from build123d import *

# Parameters (mm, degrees)
F1_DEPTH = 2.8702
F3_DEPTH = 0.8382
F4_R     = 0.127
F7_SIZE  = 0.635


with BuildPart() as f1:
    # F0 (on Front) → F1 (new body, symmetric)
    with BuildSketch(Plane.XZ):
        with BuildLine():
            Line((10.935379, 11.6078), (0.964201, 11.6078))
            ThreePointArc((0.964201, 11.6078), (8.511631, 0), (0.964201, -11.6078))
            Line((0.964201, -11.6078), (10.951463, -11.6078))
            ThreePointArc((10.951463, -11.6078), (14.342647, -7.694951), (16.055431, -2.808553))
            Line((16.055431, -2.808553), (16.055431, 6.221704))
            ThreePointArc((16.055431, 6.221704), (13.874424, 9.275049), (10.935379, 11.6078))
        make_face()
    extrude(amount=F1_DEPTH, both=True)

    # F2 (on Front) → F3 (cut, symmetric)
    with BuildSketch(Plane.XZ):
        with BuildLine():
            ThreePointArc((6.826302, 11.6078), (11.813631, 0), (6.826302, -11.6078))
            Line((6.826302, -11.6078), (10.951463, -11.6078))
            ThreePointArc((10.951463, -11.6078), (14.342647, -7.694951), (16.055431, -2.808553))
            Line((16.055431, -2.808553), (16.055431, 6.221704))
            ThreePointArc((16.055431, 6.221704), (13.874424, 9.275049), (10.935379, 11.6078))
            Line((10.935379, 11.6078), (6.826302, 11.6078))
        make_face()
    extrude(amount=F3_DEPTH, both=True, mode=Mode.SUBTRACT)

    # F4
    f4_edges = [f1.edges().sort_by_distance(p)[0] for p in [
        (11.813631, 0.8382, 0),
        (11.813631, -0.8382, 0),
    ]]
    fillet(f4_edges, radius=F4_R)

    # F5 (on Top) → F6 (revolve, cut)
    with BuildSketch(Plane.XY):
        with BuildLine():
            Line((9.46572, 2.8702), (0.964201, 2.8702))
            Line((0.964201, 2.8702), (0.964201, -2.8702))
            Line((0.964201, -2.8702), (9.46572, -2.8702))
            ThreePointArc((9.46572, -2.8702), (9.339917, -2.69481), (9.222168, -2.513915))
            ThreePointArc((9.222168, -2.513915), (9.116906, -2.335376), (9.01949, -2.152438))
            ThreePointArc((9.01949, -2.152438), (8.930418, -1.966139), (8.849484, -1.776164))
            ThreePointArc((8.849484, -1.776164), (8.777234, -1.583993), (8.713312, -1.388894))
            ThreePointArc((8.713312, -1.388894), (8.658256, -1.192864), (8.611607, -0.994664))
            ThreePointArc((8.611607, -0.994664), (8.573786, -0.796647), (8.544357, -0.59721))
            ThreePointArc((8.544357, -0.59721), (8.52352, -0.398479), (8.511016, -0.19905))
            ThreePointArc((8.511016, -0.19905), (8.506865, 0), (8.511016, 0.19905))
            ThreePointArc((8.511016, 0.19905), (8.52352, 0.398479), (8.544357, 0.59721))
            ThreePointArc((8.544357, 0.59721), (8.573786, 0.796647), (8.611607, 0.994664))
            ThreePointArc((8.611607, 0.994664), (8.658256, 1.192864), (8.713312, 1.388894))
            ThreePointArc((8.713312, 1.388894), (8.777234, 1.583993), (8.849484, 1.776164))
            ThreePointArc((8.849484, 1.776164), (8.930418, 1.966139), (9.01949, 2.152438))
            ThreePointArc((9.01949, 2.152438), (9.116906, 2.335376), (9.222168, 2.513915))
            ThreePointArc((9.222168, 2.513915), (9.339917, 2.69481), (9.46572, 2.8702))
        make_face()
        with BuildLine():
            Line((9.322597, 2.286), (9.222168, 2.513915))
            ThreePointArc((9.222168, 2.513915), (9.116906, 2.335376), (9.01949, 2.152438))
            Line((9.01949, 2.152438), (9.322597, 2.286))
        make_face()
        with BuildLine():
            Line((9.138426, 1.932211), (9.01949, 2.152438))
            ThreePointArc((9.01949, 2.152438), (8.930418, 1.966139), (8.849484, 1.776164))
            Line((8.849484, 1.776164), (9.138426, 1.932211))
        make_face()
        with BuildLine():
            ThreePointArc((9.01949, -2.152438), (9.116906, -2.335376), (9.222168, -2.513915))
            Line((9.222168, -2.513915), (9.322597, -2.286))
            Line((9.322597, -2.286), (9.01949, -2.152438))
        make_face()
        with BuildLine():
            Line((8.985791, 1.563716), (8.849484, 1.776164))
            ThreePointArc((8.849484, 1.776164), (8.777234, 1.583993), (8.713312, 1.388894))
            Line((8.713312, 1.388894), (8.985791, 1.563716))
        make_face()
        with BuildLine():
            ThreePointArc((8.849484, -1.776164), (8.930418, -1.966139), (9.01949, -2.152438))
            Line((9.01949, -2.152438), (9.138426, -1.932211))
            Line((9.138426, -1.932211), (8.849484, -1.776164))
        make_face()
        with BuildLine():
            Line((8.865852, 1.183321), (8.713312, 1.388894))
            ThreePointArc((8.713312, 1.388894), (8.658256, 1.192864), (8.611607, 0.994664))
            Line((8.611607, 0.994664), (8.865852, 1.183321))
        make_face()
        with BuildLine():
            ThreePointArc((8.713312, -1.388894), (8.777234, -1.583993), (8.849484, -1.776164))
            Line((8.849484, -1.776164), (8.985791, -1.563716))
            Line((8.985791, -1.563716), (8.713312, -1.388894))
        make_face()
        with BuildLine():
            Line((8.779524, 0.793919), (8.611607, 0.994664))
            ThreePointArc((8.611607, 0.994664), (8.573786, 0.796647), (8.544357, 0.59721))
            Line((8.544357, 0.59721), (8.779524, 0.793919))
        make_face()
        with BuildLine():
            ThreePointArc((8.611607, -0.994664), (8.658256, -1.192864), (8.713312, -1.388894))
            Line((8.713312, -1.388894), (8.865852, -1.183321))
            Line((8.865852, -1.183321), (8.611607, -0.994664))
        make_face()
        with BuildLine():
            Line((8.727463, 0.398476), (8.544357, 0.59721))
            ThreePointArc((8.544357, 0.59721), (8.52352, 0.398479), (8.511016, 0.19905))
            Line((8.511016, 0.19905), (8.727463, 0.398476))
        make_face()
        with BuildLine():
            ThreePointArc((8.544357, -0.59721), (8.573786, -0.796647), (8.611607, -0.994664))
            Line((8.611607, -0.994664), (8.779524, -0.793919))
            Line((8.779524, -0.793919), (8.544357, -0.59721))
        make_face()
        with BuildLine():
            Line((8.710065, 0), (8.511016, 0.19905))
            ThreePointArc((8.511016, 0.19905), (8.506865, 0), (8.511016, -0.19905))
            Line((8.511016, -0.19905), (8.710065, 0))
        make_face()
        with BuildLine():
            ThreePointArc((8.511016, -0.19905), (8.52352, -0.398479), (8.544357, -0.59721))
            Line((8.544357, -0.59721), (8.727463, -0.398476))
            Line((8.727463, -0.398476), (8.511016, -0.19905))
        make_face()
    revolve(axis=Axis((-4.188369, -0.221392, 0), (0, -1, 0)), mode=Mode.SUBTRACT)

    # F7
    f7_edges = [f1.edges().sort_by_distance(p)[0] for p in [
        (16.055431, -0.8382, 1.706576),
        (16.055431, 0.8382, 1.706576),
    ]]
    chamfer(f7_edges, length=F7_SIZE)


solid = f1.part
Design review of the part built by this model. Coordinates are the model's own, in mm. A direction names the side the tool comes from. Round coordinates to 2 decimals unless told otherwise and drop trailing zeros. Loops run counter-clockwise (first coordinate to the right, second up) from the corner with the lowest first, then second, coordinate; pieces in that order, holes last. Notation, with made-up numbers: (-20, -10.75) - (3, -10.75) arc R17 cw to (3, -3.75) - close; hole circle Ø7 at (82.5, 82). An arc over 180 degrees is marked (long way). One line per item, written item: value. Start each with the question number.
1) To check wall thickness, follow L1, parallel to Y at x = 12.5, z = 0.5; L2, parallel to Z at x = 7, y = -1.75; L3, parallel to Z at x = 7, y = 0.1. State the ranges of each line that lie inside material, in increasing order. Write a range as from..to.
2) For faces 5 (the flat face through (12.1, -0.838, 0.2)), 6 (the flat face through (16.055, 2, 2)), list the 3-axis set-ups (+Z, -Z, +X, -X, +Y, -Y) from which the entire face can be reached by the end or side of a thin tool; tool diameter is ignored.
3) Draft analysis for pull direction Z (two halves, no side actions). For faces 1 (the flat face through (11, 2.87, 0)), 2 (the flat face through (6, 0, -11.608)), 3 (the conical face through (8.659, -0.694, -0.206)), 4 (the conical face through (8.74, -1.09, -0.21)), state which applies: +Z half, -Z half, draft (parallel to the pull), parting line (faces both ways), or undercut.
4) Consider section A-A on x = 12.25. Give the boundary of the cut face in (y, z), then the cut area to 3 significant figures.
Reported:
1. L1: y = -2.87..-0.84, 0.84..2.87
1. L2: z = -11.61..-6.73, 6.73..11.61
1. L3: z = -11.44..-6.21, 6.21..11.44
2. face 5: +X
2. face 6: +Z, -Z, +X, +Y, -Y
3. face 1: draft
3. face 2: -Z half
3. face 3: undercut
3. face 4: undercut
4. outline: (-2.87, -10.44) - (-0.84, -10.44) - (-0.84, 10.73) - (-2.87, 10.73) - close; (0.84, -10.44) - (2.87, -10.44) - (2.87, 10.73) - (0.84, 10.73) - close
4. area: 86.0 mm^2
